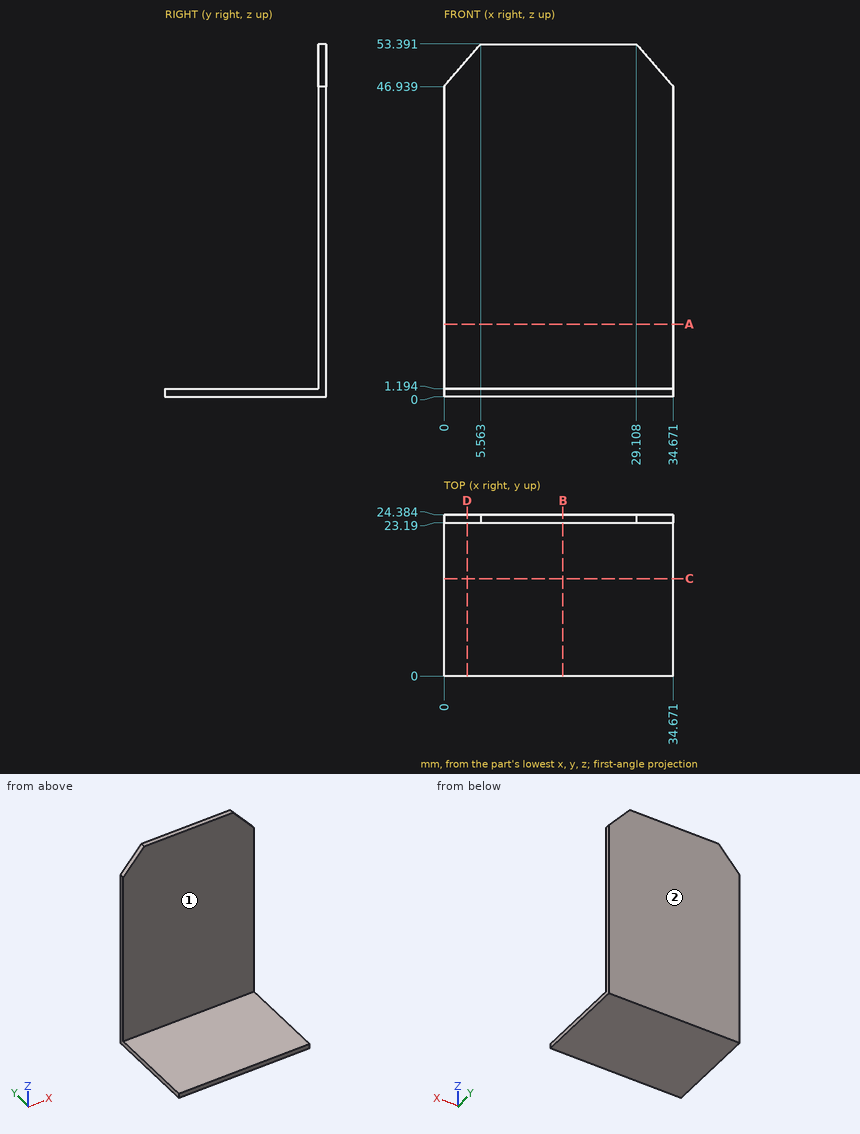
Drawing for the job (mm, zero at the part's lowest x, y, z). A direction names the side the tool comes from. Coordinates: 2 decimals unless noted, no trailing zeros. Write each loop counter-clockwise with the first axis right and the second up, starting at its lowest first coordinate (ties: lowest second). Pieces come first, ordered by that corner, then holes. Notation, with made-up numbers: (42, -15.5) -> (92, -15.5) arc R33 ccw to (92, 20.5) -> close; hole circle Ø7 at (55, -35). An arc over 180 degrees is marked (long way). One line per item, written item: value. Start each with the question number.
1) Slice it at D-D on x = 3.5. Write the cut outline in (y, z).
2) Probe probe 1 along Z at (x, y) = (20.5, 7.5); probe 2 along Y at (x, z) = (15.5, 11). List the from-to ranges inside material, lowest first.
3) Slice it at B-B on x = 18. Write the cut outline in (y, z).
4) Which spindle directions (+Z, -Z, +X, -X, +Y, -Y) get a long thin tool onto all of the face, cutting with end or side? Do the marked faces 1 and 2. Say none if no direction does.
5) Flat gauge pins, fed straight in: pin 1 Ø17.5 at (x, z) = (19, 27) entering from -Y; pin 2 Ø11.5 at (x, y) = (18.5, 6.5) entering from +Z; pin 3 Ø10 at (y, z) = (15, 40.5) entering from -X. Where does each tip first touch, or does it go through?
6) Slice it at A-A on z = 11. Write the cut outline in (x, y).
7) Slice it at C-C on y = 14.75. Write the cut outline in (x, z).
Answers follow:
1. outline: (0, 0) -> (24.38, 0) -> (24.38, 51) -> (23.19, 51) -> (23.19, 1.19) -> (0, 1.19) -> close
2. probe 1: 0 to 1.19
2. probe 2: 23.19 to 24.38
3. outline: (0, 0) -> (24.38, 0) -> (24.38, 53.39) -> (23.19, 53.39) -> (23.19, 1.19) -> (0, 1.19) -> close
4. face 1: +Z, +X, -X, -Y
4. face 2: +Z, -Z, +X, -X, +Y
5. pin 1: y = 23.19
5. pin 2: z = 1.19
5. pin 3: through
6. outline: (0, 23.19) -> (34.67, 23.19) -> (34.67, 24.38) -> (0, 24.38) -> close
7. outline: (0, 0) -> (34.67, 0) -> (34.67, 1.19) -> (0, 1.19) -> close
